from build123d import *

# Parameters (mm, degrees)
F1_DEPTH = 6
F3_DEPTH = 3
F5_DEPTH = 25


with BuildPart() as f1:
    # F0 (on Top) → F1 (new body)
    with BuildSketch(Plane.XY):
        with BuildLine():
            Line((0, 85), (-50, 85))
            ThreePointArc((-50, 85), (-78.284271, 73.284271), (-90, 45))
            Line((-90, 45), (-90, -45))
            ThreePointArc((-90, -45), (-78.284271, -73.284271), (-50, -85))
            Line((-50, -85), (50, -85))
            ThreePointArc((50, -85), (78.284271, -73.284271), (90, -45))
            Line((90, -45), (90, 0))
            Line((90, 0), (0, 0))
            Line((0, 0), (0, 85))
        make_face()
        with BuildLine():
            Line((50, 85), (0, 85))
            Line((0, 85), (0, 0))
            Line((0, 0), (90, 0))
            Line((90, 0), (90, 45))
            ThreePointArc((90, 45), (78.284271, 73.284271), (50, 85))
        make_face()
    extrude(amount=F1_DEPTH)

    # F2 (on face) → F3 (cut)
    with BuildSketch(Plane.XY.offset(6)):
        with BuildLine():
            Line((-75.375, 31.06), (-48.066738, 31.06))
            ThreePointArc((-48.066738, 31.06), (-3.825, 50), (-48.066738, 68.94))
            Line((-48.066738, 68.94), (-75.375, 68.94))
            Line((-75.375, 68.94), (-75.375, 31.06))
        make_face()
        with BuildLine():
            ThreePointArc((-45.939166, 63.94), (-8.825, 50), (-45.939166, 36.06))
            Line((-45.939166, 36.06), (-70.375, 36.06))
            Line((-70.375, 36.06), (-70.375, 63.94))
            Line((-70.375, 63.94), (-45.939166, 63.94))
        make_face(mode=Mode.SUBTRACT)
        with BuildLine():
            Line((9.625, 31.06), (36.933262, 31.06))
            ThreePointArc((36.933262, 31.06), (81.175, 50), (36.933262, 68.94))
            Line((36.933262, 68.94), (9.625, 68.94))
            Line((9.625, 68.94), (9.625, 31.06))
        make_face()
        with BuildLine():
            Line((9.625, -33.94), (36.933262, -33.94))
            ThreePointArc((36.933262, -33.94), (81.175, -15), (36.933262, 3.94))
            Line((36.933262, 3.94), (9.625, 3.94))
            Line((9.625, 3.94), (9.625, -33.94))
        make_face()
        with BuildLine():
            Line((-75.375, -33.94), (-48.066738, -33.94))
            ThreePointArc((-48.066738, -33.94), (-3.825, -15), (-48.066738, 3.94))
            Line((-48.066738, 3.94), (-75.375, 3.94))
            Line((-75.375, 3.94), (-75.375, -33.94))
        make_face()
        with BuildLine():
            Line((-70.375, 36.06), (-45.939166, 36.06))
            ThreePointArc((-45.939166, 36.06), (-8.825, 50), (-45.939166, 63.94))
            Line((-45.939166, 63.94), (-70.375, 63.94))
            Line((-70.375, 63.94), (-70.375, 36.06))
        make_face()
    extrude(amount=-F3_DEPTH, mode=Mode.SUBTRACT)

    # F4 (on face) → F5 (cut)
    with BuildSketch(Plane.XY.offset(6)):
        with BuildLine():
            ThreePointArc((17.5, -55), (16.035534, -51.464466), (12.5, -50))
            Line((12.5, -50), (-12.5, -50))
            ThreePointArc((-12.5, -50), (-16.035534, -51.464466), (-17.5, -55))
            Line((-17.5, -55), (-17.5, -70))
            ThreePointArc((-17.5, -70), (-16.035534, -73.535534), (-12.5, -75))
            Line((-12.5, -75), (12.5, -75))
            ThreePointArc((12.5, -75), (16.035534, -73.535534), (17.5, -70))
            Line((17.5, -70), (17.5, -55))
        make_face()
    extrude(amount=-F5_DEPTH, mode=Mode.SUBTRACT)


solid = f1.part
Design review of the part built by this model. Coordinates are the model's own, in mm. A direction names the side the tool comes from. Round coordinates to 2 decimals unless told otherwise and drop trailing zeros. Write each loop counter-clockwise with the first axis right and the second up, starting at its lowest first coordinate (ties: lowest second). Pieces come first, ordered by that corner, then holes. Notation, with made-up numbers: (31.25, 46) -> (36.25, 46) arc R30 cw to (36.25, 68) -> close; hole circle Ø6 at (57, -5.75). An arc over 180 degrees is marked (long way). One line per item, written item: value. Start each with the question number.
Q1. Insertion check: P1, Ø2.5, axis at x = -63.5, z = 4.5, coming from the -Y side; P2, Ø0.9, axis at x = -63.5, z = 5, coming from the -Y side; P3, Ø2.5, axis at y = 54, z = 5, coming from the +X side. Each pin has a flat end and moves straight along its axis. Give the tip position at first contact, or say it passes through.
Q2. Add section D-D (x = -30). Give the boundary of the cut face in (y, z) (3 decimals), then the cut area to 3 significant figures.
Q3. Add section C-C (y = -52.5). Give the boundary of the cut face in (x, z).
Q4. Tool access review of faces 4 (the face through (-1, 1, 6)), 5 (the face through (0, -75, 3)), 6 (the face through (81.16, -15.85, 4.52)): name each direction out of +Z, -Z, +X, -X, +Y, -Y from which nothing blocks a thin tool from reaching the whole face with its end or side.
Q5. The part is to be moulded in two halves that separate along X. For faces 1 (the face through (77.972, -73.594, 2.958)), 2 (the face through (-1, -85, 3)), 3 (the face through (-17.5, -62, 3)), say which applies: pulls with the +X half, pulls with the -X half, needs draft (parallel to the pull), parting line crosses it, or undercut.
Q6. Add section A-A (x = 2.5). Give the boundary of the cut face in (y, z).
Q7. Add section B-B (z = 1.5). Give the boundary of the cut face in (x, y), then the cut area to 3 significant figures.
Q8. To check wall thickness, follow probe 1 along Y at (x, z) = (-30, 4.95) (3 decimals); probe 2 along X at (y, z) = (3, 4.65) (3 decimals); probe 3 along Y at (x, z) = (55, 5.05) (3 decimals). State the ranges of each line that lie inside material, in increasing order.
Response:
1. P1: stops at y = -83.08
1. P2: stops at y = -82.81
1. P3: stops at x = 89.24
2. outline: (-85, 0) -> (85, 0) -> (85, 6) -> (76.175, 6) -> (76.175, 3) -> (23.825, 3) -> (23.825, 6) -> (11.175, 6) -> (11.175, 3) -> (-41.175, 3) -> (-41.175, 6) -> (-85, 6) -> close
2. area: 706 mm^2
3. outline: (-89.29, 0) -> (-16.83, 0) -> (-16.83, 6) -> (-89.29, 6) -> close; (16.83, 0) -> (89.29, 0) -> (89.29, 6) -> (16.83, 6) -> close
4. face 4: +Z, +X, -X, +Y, -Y
4. face 5: +Z, -Z
4. face 6: +Z
5. face 1: pulls with the +X half
5. face 2: needs draft
5. face 3: undercut
6. outline: (-85, 0) -> (-75, 0) -> (-75, 6) -> (-85, 6) -> close; (-50, 0) -> (85, 0) -> (85, 6) -> (-50, 6) -> close
7. outline: (-90, -45) arc R40 ccw to (-50, -85) -> (50, -85) arc R40 ccw to (90, -45) -> (90, 45) arc R40 ccw to (50, 85) -> (-50, 85) arc R40 ccw to (-90, 45) -> close; hole (-17.5, -70) arc R5 ccw to (-12.5, -75) -> (12.5, -75) arc R5 ccw to (17.5, -70) -> (17.5, -55) arc R5 ccw to (12.5, -50) -> (-12.5, -50) arc R5 ccw to (-17.5, -55) -> close
7. area: 28,400 mm^2
8. probe 1: y = -85 to -41.175, 11.175 to 23.825, 76.175 to 85
8. probe 2: x = -90 to -75.375, -10.997 to 9.625, 74.003 to 90
8. probe 3: y = -84.686 to -41.175, 11.175 to 23.825, 76.175 to 84.686
